Read the model definition and answer for the solid it produces. Units are mm, in the model's axes. A direction names the side the tool comes from. Coordinates: 2 decimals unless noted, no trailing zeros. Order: outer loops, then holes, each group sorted by start corner. A loop starts at its lowest first (then second) coordinate and runs counter-clockwise, first axis right, second up. Notation, with made-up numbers: M 9.25,-4 L 25.25,-4 A18 ccw 25.25,27 Z; hole C 84.25,85.5 d7. An arc over 180 degrees is marked long. One line per question, with ' | ' between items. Start each with the question number.
1) Consider probe 1 along X at (y, z) = (6.5, -4.5); probe 2 along Y at (x, z) = (-33, 12); probe 3 along X at (y, z) = (-4.5, 0). Determine where each line is inside the solid, lowest interval first.
2) The mould has two halves that part along X. Classify faces 1 (the face through (-9, 0, 28)), 2 (the face through (-12.9, -7.46, 17.58)), 3 (the face through (6.85, 4.93, 27.02)), 4 (the face through (-22.05, 0.24, -28.76)): +X half, -X half, draft (parallel to the pull), parting line (faces both ways), or undercut.
3) Find section B-B, the plane y = -8.5. Write down the section's boundary in (x, z).
4) Find section A-A, the plane x = 0. Write down the section's boundary in (y, z).
5) Given P1, Ø10, axis at x = -3, y = 5, coming from the +Z side; P2, Ø12, axis at x = -17, y = 4, coming from the -Z side; P3, Ø9, axis at x = -26.7, z = 19.4, coming from the -Y side; P4, Ø1, axis at y = -6, z = -15.5, coming from the -X side, each flat-ended and moving along its own axis, determine where each tip first touches the part or whether it passes through.
6) Find section C-C, the plane x = 11.75. Count the separate pieces of the cut face and the enclosed holes in it, plus the area to 3 significant figures.
7) A tool of negligible diameter and unlimited length cuts with its end or side. For faces 5 (the face through (-7.086, -6.451, -17.089)), 6 (the face through (18, -10, -6)), 7 (the face through (25, 0, 19)), from which of +Z, -Z, +X, -X, +Y, -Y can it reach the whole face along a straight path? Write none if from no direction.
from build123d import *

# Parameters (mm, degrees)
SKETCH1_R                = 41
SKETCH1_R_2              = 5.5
SKETCH1_R_3              = 25
BOSS_EXTRUDE1_DEPTH      = 10
SKETCH2_R                = 25
SKETCH2_R_2              = 22.5
BOSS_EXTRUDE2_DEPTH      = 10
BOSS_EXTRUDE4_DEPTH      = 10
BOSS_EXTRUDE4_DEPTH_BACK = 10
SKETCH4_R                = 27.5
SKETCH4_R_2              = 19.5
SKETCH4_R_3              = 3
BOSS_EXTRUDE5_START      = -10
BOSS_EXTRUDE5_DEPTH      = 10
BOSS_EXTRUDE6_START      = -10
SKETCH6_R                = 3
BOSS_EXTRUDE6_DEPTH      = 5
CHAMFER2_SIZE            = 5
BOSS_EXTRUDE7_START      = -20
SKETCH7_R                = 19.5
SKETCH7_R_2              = 18.5
BOSS_EXTRUDE7_DEPTH      = 20
SKETCH8_R                = 18.5
SKETCH8_R_2              = 16
BOSS_EXTRUDE8_DEPTH      = 13
CHAMFER4_SIZE            = 10


with BuildPart() as part:
    # Sketch1 → Boss-Extrude1 (new body)
    with BuildSketch(Plane(origin=(0, 0, 0), x_dir=(1, 0, 0), z_dir=(0, 1, 0))):
        with Locations(Location((0, 0, 0), (0, 0, 270))):
            Circle(SKETCH1_R)
        with Locations(Location((33, 0, 0), (0, 0, 270))):
            Circle(SKETCH1_R_2, mode=Mode.SUBTRACT)
        with Locations(Location((10.197560814, -31.384865038, 0), (0, 0, 270))):
            Circle(SKETCH1_R_2, mode=Mode.SUBTRACT)
        with Locations(Location((-26.697560814, -19.396913326, 0), (0, 0, 270))):
            Circle(SKETCH1_R_2, mode=Mode.SUBTRACT)
        with Locations(Location((-26.697560814, 19.396913326, 0), (0, 0, 270))):
            Circle(SKETCH1_R_2, mode=Mode.SUBTRACT)
        with Locations(Location((10.197560814, 31.384865038, 0), (0, 0, 270))):
            Circle(SKETCH1_R_2, mode=Mode.SUBTRACT)
        with Locations(Location((0, 0, 0), (0, 0, 270))):
            Circle(SKETCH1_R_3, mode=Mode.SUBTRACT)
    extrude(amount=BOSS_EXTRUDE1_DEPTH)

    # Sketch2 → Boss-Extrude2 (add)
    with BuildSketch(Plane.XZ):
        Circle(SKETCH2_R)
        with Locations(Location((0, 0, 0), (0, 0, 270))):
            Circle(SKETCH2_R_2, mode=Mode.SUBTRACT)
    extrude(amount=-BOSS_EXTRUDE2_DEPTH)

    # Sketch4 → Boss-Extrude4 (add, two sides: drawn at the far end of the back side and taken through both)
    with BuildSketch(Plane.XZ.offset(-BOSS_EXTRUDE4_DEPTH_BACK)):
        with Locations(Location((0, 0, 0), (0, 0, 270))):
            Circle(SKETCH4_R)
        with Locations(Location((0, 0, 0), (0, 0, 270))):
            Circle(SKETCH4_R_2, mode=Mode.SUBTRACT)
        with Locations(Location((23.5, 0, 0), (0, 0, 270))):
            Circle(SKETCH4_R_3, mode=Mode.SUBTRACT)
        with Locations(Location((11.75, -20.351596989, 0), (0, 0, 270))):
            Circle(SKETCH4_R_3, mode=Mode.SUBTRACT)
        with Locations(Location((-11.75, -20.351596989, 0), (0, 0, 270))):
            Circle(SKETCH4_R_3, mode=Mode.SUBTRACT)
        with Locations(Location((-23.5, 0, 0), (0, 0, 270))):
            Circle(SKETCH4_R_3, mode=Mode.SUBTRACT)
        with Locations(Location((-11.75, 20.351596989, 0), (0, 0, 270))):
            Circle(SKETCH4_R_3, mode=Mode.SUBTRACT)
        with Locations(Location((11.75, 20.351596989, 0), (0, 0, 270))):
            Circle(SKETCH4_R_3, mode=Mode.SUBTRACT)
    extrude(amount=BOSS_EXTRUDE4_DEPTH + BOSS_EXTRUDE4_DEPTH_BACK)

    # Sketch5 → Boss-Extrude5 (add)
    with BuildSketch(Plane(origin=(0, 10, 0), x_dir=(1, 0, 0), z_dir=(0, 1, 0)).offset(BOSS_EXTRUDE5_START)):
        with BuildLine():
            ThreePointArc((-13.557162741, 17.956985783), (-10.25, 17.753520778), (-8.772624493, 20.719340229))
            ThreePointArc((-8.772624493, 20.719340229), (-11.25, 19.485571585), (-13.557162741, 17.956985783))
        make_face()
        with BuildLine():
            ThreePointArc((-22.329787234, 2.762354445), (-22.5, 0), (-22.329787234, -2.762354445))
            ThreePointArc((-22.329787234, -2.762354445), (-20.5, 0), (-22.329787234, 2.762354445))
        make_face()
        with BuildLine():
            ThreePointArc((8.772624493, 20.719340229), (10.25, 17.753520778), (13.557162741, 17.956985783))
            ThreePointArc((13.557162741, 17.956985783), (11.25, 19.485571585), (8.772624493, 20.719340229))
        make_face()
        with BuildLine():
            ThreePointArc((22.329787234, 2.762354445), (20.5, 0), (22.329787234, -2.762354445))
            ThreePointArc((22.329787234, -2.762354445), (22.5, 0), (22.329787234, 2.762354445))
        make_face()
        with BuildLine():
            ThreePointArc((13.557162741, -17.956985783), (10.25, -17.753520778), (8.772624493, -20.719340229))
            ThreePointArc((8.772624493, -20.719340229), (11.25, -19.485571585), (13.557162741, -17.956985783))
        make_face()
        with BuildLine():
            ThreePointArc((-8.772624493, -20.719340229), (-10.25, -17.753520778), (-13.557162741, -17.956985783))
            ThreePointArc((-13.557162741, -17.956985783), (-11.25, -19.485571585), (-8.772624493, -20.719340229))
        make_face()
    extrude(amount=BOSS_EXTRUDE5_DEPTH)

    # Sketch6 → Boss-Extrude6 (add)
    with BuildSketch(Plane.XZ.offset(10).offset(BOSS_EXTRUDE6_START)):
        with Locations(Location((-23.5, 0, 0), (0, 0, 270))):
            Circle(SKETCH6_R)
        with Locations(Location((-11.75, 20.351596989, 0), (0, 0, 270))):
            Circle(SKETCH6_R)
        with Locations(Location((11.75, 20.351596989, 0), (0, 0, 270))):
            Circle(SKETCH6_R)
        with Locations(Location((23.5, 0, 0), (0, 0, 270))):
            Circle(SKETCH6_R)
        with Locations(Location((11.75, -20.351596989, 0), (0, 0, 270))):
            Circle(SKETCH6_R)
        with Locations(Location((-11.75, -20.351596989, 0), (0, 0, 270))):
            Circle(SKETCH6_R)
    extrude(amount=BOSS_EXTRUDE6_DEPTH)

    # Chamfer2
    # the kernel refuses this chamfer: 5 mm, written as the material it takes off along each edge
    with BuildSketch(Plane(origin=(0, 0, 0), x_dir=(0, 0, 1), z_dir=(-1, 0, 0))) as chamfer2_piece_1:
        Polygon((41, CHAMFER2_SIZE), (41 - CHAMFER2_SIZE, 0), (41, 0), align=None)
    revolve(axis=Axis((0, 0, 0), (0, 1, 0)), mode=Mode.SUBTRACT)

    # Sketch7 → Boss-Extrude7 (add)
    with BuildSketch(Plane.XZ.offset(10).offset(BOSS_EXTRUDE7_START)):
        Circle(SKETCH7_R)
        with Locations(Location((0, 0, 0), (0, 0, 270))):
            Circle(SKETCH7_R_2, mode=Mode.SUBTRACT)
    extrude(amount=BOSS_EXTRUDE7_DEPTH)

    # Sketch8 → Boss-Extrude8 (add)
    with BuildSketch(Plane(origin=(0, 10, 0), x_dir=(1, 0, 0), z_dir=(0, 1, 0))):
        with Locations(Location((0, 0, 0), (0, 0, 90))):
            Circle(SKETCH8_R)
        with Locations(Location((0, 0, 0), (0, 0, 270))):
            Circle(SKETCH8_R_2, mode=Mode.SUBTRACT)
    extrude(amount=-BOSS_EXTRUDE8_DEPTH)

    # Chamfer4
    chamfer4_edges = [part.edges().sort_by_distance(p)[0] for p in [
        (0, 10, -16),
    ]]
    chamfer(chamfer4_edges, length=CHAMFER4_SIZE)


solid = part.part
Report:
1) probe 1: x = -40.75 to -22.05, 22.05 to 29.84, 36.16 to 40.75 | probe 2: y = 0 to 10 | probe 3: x = -27.5 to -18.5, 18.5 to 27.5
2) face 1: draft | face 2: undercut | face 3: undercut | face 4: parting line
3) outline: C 0,0 d55; hole C -23.5,0 d6; hole C 0,0 d37; hole C -11.75,-20.35 d6; hole C -11.75,20.35 d6; hole C 11.75,-20.35 d6; hole C 11.75,20.35 d6; hole C 23.5,0 d6
4) outline: M -10,-27.5 L 0,-27.5 L 0,-36 L 5,-41 L 10,-41 L 10,-26 L 0,-16 L -3,-16 L -3,-18.5 L -10,-18.5 Z; M -10,18.5 L -3,18.5 L -3,16 L 0,16 L 10,26 L 10,41 L 5,41 L 0,36 L 0,27.5 L -10,27.5 Z
5) P1: stops at z = 41 | P2: stops at z = -39.47 | P3: passes through | P4: stops at x = -23.05
6) separate pieces: 4 | enclosed holes: 0 | area: 381 mm^2
7) face 5: -Y | face 6: +Z, -Z, +X, -X, -Y | face 7: +Z, +X, -Y
